```python
from build123d import *

# Parameters (mm, degrees)
SKETCH1_W            = 70
SKETCH1_H            = 50
BOSS_EXTRUDE1_DEPTH  = 50
SKETCH2_W            = 50
SKETCH2_H            = 10
CUT_EXTRUDE1_DEPTH   = 50
SKETCH3_W            = 50
SKETCH3_H            = 40
CUT_EXTRUDE2_DEPTH   = 40
CUT_EXTRUDE6_DEPTH   = 20
BOSS_EXTRUDE9_DEPTH  = 20
BOSS_EXTRUDE10_DEPTH = 20
SKETCH11_W           = 20
SKETCH11_H           = 20
CUT_EXTRUDE7_DEPTH   = 20
BOSS_EXTRUDE12_DEPTH = 10
BOSS_EXTRUDE13_DEPTH = 10
CUT_EXTRUDE8_DEPTH   = 68


with BuildPart() as part:
    # Sketch1 → Boss-Extrude1 (new body)
    with BuildSketch(Plane.XY):
        with Locations((35, 25)):
            Rectangle(SKETCH1_W, SKETCH1_H)
    extrude(amount=BOSS_EXTRUDE1_DEPTH)

    # Sketch2 → Cut-Extrude1 (cut)
    with BuildSketch(Plane.XY.offset(50)):
        with Locations((25, 45)):
            Rectangle(SKETCH2_W, SKETCH2_H)
    extrude(amount=-CUT_EXTRUDE1_DEPTH, mode=Mode.SUBTRACT)

    # Sketch3 → Cut-Extrude2 (cut)
    with BuildSketch(Plane.XY.offset(50)):
        with Locations((25, 20)):
            Rectangle(SKETCH3_W, SKETCH3_H)
    extrude(amount=-CUT_EXTRUDE2_DEPTH, mode=Mode.SUBTRACT)

    # Sketch8 → Cut-Extrude6 (cut)
    with BuildSketch(Plane.XY.offset(10)):
        Polygon((30, 40), (0, 20), (20, 20), (50, 40), align=None)
    extrude(amount=-CUT_EXTRUDE6_DEPTH, mode=Mode.SUBTRACT)

    # Sketch9 → Boss-Extrude9 (add)
    with BuildSketch(Plane.XY.offset(10)):
        Polygon((50, 40), (20, 20), (20, 0), (50, 0), align=None)
    extrude(amount=BOSS_EXTRUDE9_DEPTH)

    # Sketch10 → Boss-Extrude10 (add)
    with BuildSketch(Plane(origin=(-9.411764706, 14.117647059, 9.411764706), x_dir=(0.874474632, 0.403603676, 0.269069118), z_dir=(-0.48507125, 0.727606875, 0.48507125))):
        Polygon((45.069077198, 13.867504906), (67.939952194, -2.773500981), (33.6336397, -13.867504906), (10.762764704, 2.773500981), align=None)
    extrude(amount=-BOSS_EXTRUDE10_DEPTH)

    # Sketch11 → Cut-Extrude7 (cut)
    with BuildSketch(Plane.ZY.offset(-20)):
        with Locations((20, 10)):
            Rectangle(SKETCH11_W, SKETCH11_H)
    extrude(amount=CUT_EXTRUDE7_DEPTH, mode=Mode.SUBTRACT)

    # Sketch12 → Boss-Extrude12 (add)
    with BuildSketch(Plane(origin=(0, 0, 0), x_dir=(-1, 0, 0), z_dir=(0, 0, -1))):
        Polygon((-50, 40), (-20, 20), (0, 20), (-30, 40), align=None)
    extrude(amount=-BOSS_EXTRUDE12_DEPTH)

    # Sketch13 → Boss-Extrude13 (add)
    with BuildSketch(Plane(origin=(0, 40, 0), x_dir=(1, 0, 0), z_dir=(0, 1, 0))):
        Polygon((30, -10), (50, -10), (50, -30), align=None)
    extrude(amount=-BOSS_EXTRUDE13_DEPTH)

    # Sketch14 → Cut-Extrude8 (cut)
    with BuildSketch(Plane(origin=(0, 50, 0), x_dir=(1, 0, 0), z_dir=(0, 1, 0))):
        Polygon((70, -50), (50, -40), (50, -50), align=None)
    extrude(amount=-CUT_EXTRUDE8_DEPTH, mode=Mode.SUBTRACT)


solid = part.part
```
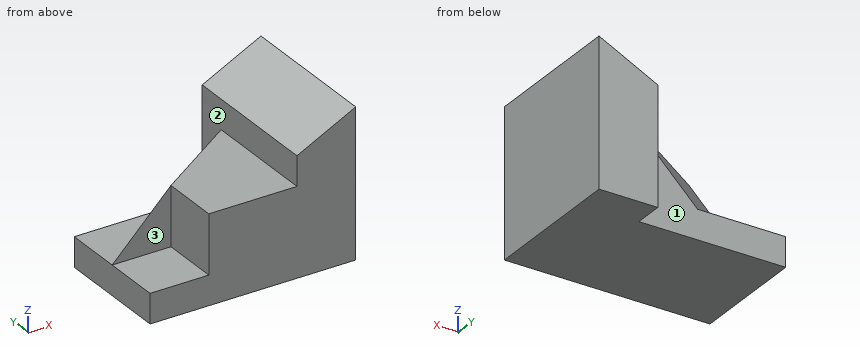
Geometry check sheet. Reference: the model listing, model coordinates, mm. Face numbers are marked on the shaded views. A direction names the side the tool comes from. Coordinates: 2 decimals unless noted, no trailing zeros. Write each loop counter-clockwise with the first axis right and the second up, starting at its lowest first coordinate (ties: lowest second). Pieces come first, ordered by that corner, then holes. Notation, with made-up numbers: M 66,53 L 93,53 A27 cw 93,88 Z; hole C -23,-13.75 d11. An arc over 180 degrees is marked long. One line per item, written item: value. Start each with the question number.
(1) Scan lines: line 1 along X through (y, z) = (4, 15); line 2 along X through (y, z) = (9.5, 40); line 3 along Z through (x, y) = (30, 9.5). Record each from-to range of solid material in increasing order. Write a range as [from, to].
(2) Sectioned sample at C-C, the plane z = 25. Enter the section's corners in (x, y).
(3) Tool access check on the marked faces 1, 2 and 3. Record the directions out of +Z, -Z, +X, -X, +Y, -Y that give a thin tool (end or side, any length) a straight path to the whole face; none if there is none.
(4) Sectioned sample at B-B, the plane x = 4.5. Enter the section's corners in (y, z), and give its area (3 significant figures).
(5) Sectioned sample at D-D, the plane x = 47. Enter the section's corners in (y, z), and give its area (3 significant figures).
(6) Sectioned sample at A-A, the plane y = 21. Enter the section's corners in (x, z), and give its area (3 significant figures).
(7) Depth check by flat-ended pin: pin 1 (1 mm diameter, centred on x = 24, z = 13, fed in from +Y); pin 2 (16 mm diameter, centred on y = 8, z = 24, fed in from -X); pin 3 (16 mm diameter, centred on x = 20, y = 31.5, fed in from +Z). Enter the tip coordinate at first touch or a pass-through.
Filled sheet:
1. line 1: [20, 70]
1. line 2: [50, 70]
1. line 3: [0, 30]
2. outline: M 15,20 L 20,20 L 20,0 L 70,0 L 70,50 L 50,50 L 50,40 L 45,40 Z
3. face 1: +Z, -Z, -X, +Y
3. face 2: +Z, -X, +Y
3. face 3: +Z, -X, -Y
4. outline: M 0,0 L 40,0 L 40,10 L 23,10 L 20,14.5 L 20,10 L 0,10 Z
4. area: 407 mm²
5. outline: M 0,0 L 40,0 L 40,27 L 38,30 L 0,30 Z
5. area: 1,200 mm²
6. outline: M 0,0 L 70,0 L 70,50 L 50,40 L 50,30 L 21.5,30 L 1.5,10 L 0,10 Z
6. area: 2,170 mm²
7. pin 1: y = 34.47
7. pin 2: x = 20
7. pin 3: z = 27.17
